```python
from build123d import *

# Parameters (mm, degrees)
BOSS_EXTRUDE1_DEPTH      = 11
BOSS_EXTRUDE1_DEPTH_BACK = 12
SKETCH1_W                = 9.5
SKETCH1_H                = 6.5
SKETCH2_W                = 9.5
SKETCH2_H                = 10
BOSS_EXTRUDE2_DEPTH      = 10
SKETCH3_R                = 1.5
BOSS_EXTRUDE3_DEPTH      = 3
SKETCH4_W                = 9.5
SKETCH4_H                = 6.5
BOSS_EXTRUDE4_DEPTH      = 0.5


with BuildPart() as part:
    # Sketch1 → Boss-Extrude1 (new, two sides: drawn at the far end of the back side and taken through both)
    with BuildSketch(Plane.XY.offset(-BOSS_EXTRUDE1_DEPTH_BACK)):
        Rectangle(SKETCH1_W, SKETCH1_H)
    extrude(amount=BOSS_EXTRUDE1_DEPTH + BOSS_EXTRUDE1_DEPTH_BACK)

    # Sketch2 → Boss-Extrude2 (add)
    with BuildSketch(Plane(origin=(0, 3.25, 0), x_dir=(1, 0, 0), z_dir=(0, 1, 0))):
        Rectangle(SKETCH2_W, SKETCH2_H)
    extrude(amount=BOSS_EXTRUDE2_DEPTH)

    # Sketch3 → Boss-Extrude3 (add)
    with BuildSketch(Plane(origin=(0, 0, -12), x_dir=(-1, 0, 0), z_dir=(0, 0, -1))):
        Circle(SKETCH3_R)
    extrude(amount=BOSS_EXTRUDE3_DEPTH)

    # Sketch4 → Boss-Extrude4 (add)
    with BuildSketch(Plane.XY.offset(11)):
        Rectangle(SKETCH4_W, SKETCH4_H)
    extrude(amount=BOSS_EXTRUDE4_DEPTH)


solid = part.part
```
Read the model definition and answer for the solid it produces. Units are mm, in the model's axes. A direction names the side the tool comes from. Round coordinates to 2 decimals unless told otherwise and drop trailing zeros. Write each loop counter-clockwise with the first axis right and the second up, starting at its lowest first coordinate (ties: lowest second). Pieces come first, ordered by that corner, then holes. Notation, with made-up numbers: M 2.5,19.5 L 21.5,19.5 A6 ccw 21.5,25.5 Z; hole C 88.5,-24.5 d6. An arc over 180 degrees is marked long. One line per item, written item: value.
Q1. Find section B-B on x = 0. Write down the section's boundary in (y, z).
Data:
outline: M -3.25,-12 L -1.5,-12 L -1.5,-15 L 1.5,-15 L 1.5,-12 L 3.25,-12 L 3.25,-5 L 13.25,-5 L 13.25,5 L 3.25,5 L 3.25,11.5 L -3.25,11.5 Z
Q2. Find section D-D on x = -3.5. Write down the section's boundary in (y, z).
Data:
outline: M -3.25,-12 L 3.25,-12 L 3.25,-5 L 13.25,-5 L 13.25,5 L 3.25,5 L 3.25,11.5 L -3.25,11.5 Z
Q3. Straight lines are drawn through the part: line 1 (Z direction, x = 1.75, y = 8); line 2 (Z direction, x = -1.75, y = 0.5); line 3 (Y direction, x = 2, z = 8.25). For each, find the intervals that lie inside material, in ascending order. Write a range as [from, to].
Data:
line 1: [-5, 5]
line 2: [-12, 11.5]
line 3: [-3.25, 3.25]
Q4. Find section A-A on y = 0. Write down the section's boundary in (x, z), plus the area to 3 significant figures.
Data:
outline: M -4.75,-12 L -1.5,-12 L -1.5,-15 L 1.5,-15 L 1.5,-12 L 4.75,-12 L 4.75,11.5 L -4.75,11.5 Z
area: 232 mm2
Q5. Which of the six approach directions +Z, -Z, +X, -X, +Y, -Y give full straight-line access (tool end or side, diameter ignored) to faces 1 (the flat face through (0, 8, 5)), 2 (the flat face through (0, 0, 11.5)), 3 (the cylindrical face through (1.5, 0.07, -13.48)), 4 (the flat face through (0, 3.25, -9))?
Data:
face 1: +Z, +X, -X, +Y
face 2: +Z, +X, -X, +Y, -Y
face 3: -Z
face 4: -Z, +X, -X, +Y
Q6. A flat-ended cylindrical pin translates along its axis: pin 1 Ø5.5 at (x, z) = (1.5, -9.5) entering from +Y. Find the tip coordinate at first contact, or state that the pin passes through.
Data:
pin 1: y = 3.25
Q7. Find section C-C on z = 8. Write down the section's boundary in (x, y).
Data:
outline: M -4.75,-3.25 L 4.75,-3.25 L 4.75,3.25 L -4.75,3.25 Z
